```python
from build123d import *

# Parameters (mm, degrees)
SKETCH2_R               = 43.815
SKETCH2_R_2             = 40
BASE_CYLINDER_DEPTH     = 381
SKETCH3_R               = 56.35625
SKETCH3_R_2             = 40
AFT_FLANGE_DEPTH        = 9.525
SKETCH6_R               = 46.9011
SKETCH6_R_2             = 44.2849
AFT_O_RING_DEPTH        = 1.9812
SKETCH33_R              = 45.72
SKETCH33_R_2            = 43.815
CRITICALBOSS_DEPTH      = 31.75
FILLET1_R               = 2.54
BOLT_CIRCLE_D           = 4.0386
HOLE1_D                 = 2.38125
HOLE1_CBORE_D           = 4.7625
HOLE1_CBORE_DEPTH       = 4.7625
F_3_8_24_TAPPED_HOLE1_D = 8.4328
FILLET1_OF_MIRROR1_R    = 2.54


with BuildPart() as part:
    # Sketch2 → Base Cylinder (new body)
    with BuildSketch(Plane(origin=(0, 0, 0), x_dir=(1, 0, 0), z_dir=(0, 1, 0))):
        with Locations(Location((0, 0, 0), (0, 0, 270))):
            Circle(SKETCH2_R)
        with Locations(Location((0, 0, 0), (0, 0, 270))):
            Circle(SKETCH2_R_2, mode=Mode.SUBTRACT)
    extrude(amount=BASE_CYLINDER_DEPTH)

    # Sketch3 → Aft Flange (add)
    with BuildSketch(Plane.XZ):
        with Locations(Location((0, 0, 0), (0, 0, 270))):
            Circle(SKETCH3_R)
        with Locations(Location((0, 0, 0), (0, 0, 90))):
            Circle(SKETCH3_R_2, mode=Mode.SUBTRACT)
    aft_flange = extrude(amount=-AFT_FLANGE_DEPTH)

    # Sketch6 → Aft O-Ring (cut)
    with BuildSketch(Plane.XZ):
        with Locations(Location((0, 0, 0), (0, 0, 270))):
            Circle(SKETCH6_R)
        with Locations(Location((0, 0, 0), (0, 0, 270))):
            Circle(SKETCH6_R_2, mode=Mode.SUBTRACT)
    aft_o_ring = extrude(amount=-AFT_O_RING_DEPTH, mode=Mode.SUBTRACT)

    # Sketch33 → CriticalBoss (add)
    with BuildSketch(Plane(origin=(0, 9.525, 0), x_dir=(1, 0, 0), z_dir=(0, 1, 0))):
        with Locations(Location((0, 0, 0), (0, 0, 90))):
            Circle(SKETCH33_R)
        with Locations(Location((0, 0, 0), (0, 0, 270))):
            Circle(SKETCH33_R_2, mode=Mode.SUBTRACT)
    criticalboss = extrude(amount=CRITICALBOSS_DEPTH)

    # Fillet1
    # the kernel refuses this fillet: 2.54 mm, written as the material it adds along each edge
    with BuildSketch(Plane(origin=(0, 9.525, 0), x_dir=(0, 0, -1), z_dir=(1, 0, 0))) as fillet1_piece_1:
        with BuildLine():
            CenterArc((45.72 + FILLET1_R, FILLET1_R), FILLET1_R, 180, 90)
            Line((45.72, FILLET1_R), (45.72 - FILLET1_R * 0.02, FILLET1_R))
            Line((45.72 - FILLET1_R * 0.02, FILLET1_R), (45.72 - FILLET1_R * 0.02, -FILLET1_R * 0.02))
            Line((45.72 - FILLET1_R * 0.02, -FILLET1_R * 0.02), (45.72 + FILLET1_R, -FILLET1_R * 0.02))
            Line((45.72 + FILLET1_R, -FILLET1_R * 0.02), (45.72 + FILLET1_R, 0))
        make_face()
    revolve(axis=Axis((0, 9.525, 0), (0, 1, 0)))
    with BuildSketch(Plane(origin=(0, 41.275, 0), x_dir=(0, 0, 1), z_dir=(-1, 0, 0))) as fillet1_piece_2:
        with BuildLine():
            CenterArc((46.355, 2.459344425), FILLET1_R, 180, 75.522487814)
            Line((43.815, 2.459344425), (43.7642, 2.459344425))
            Line((43.7642, 2.459344425), (43.7642, 0))
            Line((43.7642, 0), (43.815, -0.0508))
            ThreePointArc((43.815, -0.0508), (44.7675, -0.0508), (45.7073, -0.049186888))
            Line((45.7073, -0.049186888), (45.72, 0))
        make_face()
    revolve(axis=Axis((0, 41.275, 0), (0, 1, 0)))

    # Bolt Circle (through all)
    with Locations(Plane(origin=(0, 0, 0), x_dir=(-1, 0, 0), z_dir=(0, -1, 0))):
        with Locations((-25.81275, -44.708994483), (-44.708994483, -25.81275), (-51.6255, 0), (-44.708994483, 25.81275), (-25.81275, 44.708994483), (0, 51.6255), (25.81275, 44.708994483), (44.708994483, 25.81275), (51.6255, 0), (44.708994483, -25.81275), (25.81275, -44.708994483), (0, -51.6255)):
            bolt_circle = Hole(BOLT_CIRCLE_D / 2)

    # Hole1 (through all)
    with Locations(Plane(origin=(0, 0, 0), x_dir=(-1, 0, 0), z_dir=(0, -1, 0))):
        with Locations((49.866403745, 13.361662613), (-49.866403745, -13.361662613)):
            hole1 = CounterBoreHole(HOLE1_D / 2, HOLE1_CBORE_D / 2, HOLE1_CBORE_DEPTH)

    # Sketch44 → 1/8 NPT Tapped ThermocoupleHole (revolve, cut)
    with BuildSketch(Plane(origin=(0, 19.05, -45.72), x_dir=(0, 1, 0), z_dir=(1, 0, 0))):
        Polygon((0, 0), (0, 14.213468714), (4.2164, 11.68), (4.2164, 6.86), (4.537404713, 6.86), (4.7428023, 0), align=None)
    revolve(axis=Axis((0, 19.05, -52.07), (0, 0, 1)), mode=Mode.SUBTRACT)

    # 3/8-24 Tapped Hole1 (through all)
    with Locations(Plane.XY.offset(45.72)):
        with Locations((0, 19.05)):
            Hole(F_3_8_24_TAPPED_HOLE1_D / 2)

    # Mirror1: Aft Flange, Aft O-Ring, CriticalBoss, Bolt Circle, Hole1 across plane
    add(aft_flange.mirror(Plane.ZX.offset(190.5)))
    add(aft_o_ring.mirror(Plane.ZX.offset(190.5)), mode=Mode.SUBTRACT)
    add(criticalboss.mirror(Plane.ZX.offset(190.5)))
    add(bolt_circle.mirror(Plane.ZX.offset(190.5)), mode=Mode.SUBTRACT)
    add(hole1.mirror(Plane.ZX.offset(190.5)), mode=Mode.SUBTRACT)

    # Fillet1 of Mirror1
    # the kernel refuses this fillet: 2.54 mm, written as the material it adds along each edge
    with BuildSketch(Plane(origin=(0, 371.475, 0), x_dir=(0, 0, -1), z_dir=(1, 0, 0))) as fillet1_of_mirror1_piece_1:
        with BuildLine():
            CenterArc((45.72 + FILLET1_OF_MIRROR1_R, -FILLET1_OF_MIRROR1_R), FILLET1_OF_MIRROR1_R, 90, 90)
            Line((45.72 + FILLET1_OF_MIRROR1_R, 0), (45.72 + FILLET1_OF_MIRROR1_R, FILLET1_OF_MIRROR1_R * 0.02))
            Line((45.72 + FILLET1_OF_MIRROR1_R, FILLET1_OF_MIRROR1_R * 0.02), (45.72 - FILLET1_OF_MIRROR1_R * 0.02, FILLET1_OF_MIRROR1_R * 0.02))
            Line((45.72 - FILLET1_OF_MIRROR1_R * 0.02, FILLET1_OF_MIRROR1_R * 0.02), (45.72 - FILLET1_OF_MIRROR1_R * 0.02, -FILLET1_OF_MIRROR1_R))
            Line((45.72 - FILLET1_OF_MIRROR1_R * 0.02, -FILLET1_OF_MIRROR1_R), (45.72, -FILLET1_OF_MIRROR1_R))
        make_face()
    revolve(axis=Axis((0, 371.475, 0), (0, 1, 0)))
    with BuildSketch(Plane(origin=(0, 339.725, 0), x_dir=(0, 0, 1), z_dir=(-1, 0, 0))) as fillet1_of_mirror1_piece_2:
        with BuildLine():
            CenterArc((46.355, -2.459344425), FILLET1_OF_MIRROR1_R, 104.477512186, 75.522487814)
            Line((45.72, 0), (45.7073, 0.049186888))
            ThreePointArc((45.7073, 0.049186888), (44.7675, 0.0508), (43.815, 0.0508))
            Line((43.815, 0.0508), (43.7642, 0))
            Line((43.7642, 0), (43.7642, -2.459344425))
            Line((43.7642, -2.459344425), (43.815, -2.459344425))
        make_face()
    revolve(axis=Axis((0, 339.725, 0), (0, 1, 0)))


solid = part.part
```
The listing builds one solid part. Answer for the finished solid, in the listing's coordinates (mm). A direction names the side the tool comes from. Coordinates: 2 decimals unless noted, no trailing zeros. Write each loop counter-clockwise with the first axis right and the second up, starting at its lowest first coordinate (ties: lowest second). Pieces come first, ordered by that corner, then holes.
Q1. The mould has two halves that part along X. Classify faces 6 (the flat face through (-23, 0, 33)), 7 (the cylindrical face through (-16.96, 380.02, -40.91)), 8 (the cylindrical face through (-21.58, 376.3, -52.06)): released by +X, released by -X, zero draft, split by the parting line, or undercut.
Returned:
face 6: zero draft
face 7: undercut
face 8: split by the parting line
Q2. Find the intervals of material crossed by line 1 along X through (y, z) = (318.5, 1); line 2 along Y through (x, z) = (-49, -17) (3 decimals); line 3 along Z through (x, y) = (-3, 326.5), in increasing order.
Returned:
line 1: x = -43.8 to -39.99, 39.99 to 43.8
line 2: y = 0 to 9.525, 371.475 to 381
line 3: z = -43.71 to -39.89, 39.89 to 43.71
Q3. Given P1, Ø2.5, axis at x = 50, z = 14, coming from the +Y side; P2, Ø8, axis at y = 291.5, z = 5, coming from the -X side; P3, Ø1.5, axis at x = 12.5, y = 241, coming from the -Z side, each flat-ended and moving along its own axis, determine where each tip first touches the part or whether it passes through.
Returned:
P1: stops at y = 376.24
P2: stops at x = -43.8
P3: stops at z = -42.21
Q4. Section B-B, the plane y = 265.5 is taken. Write down the section's boundary in (x, z) (3 decimals), then the cut area to 3 significant figures.
Returned:
outline: circle Ø87.63 at (0, 0); hole circle Ø80 at (0, 0)
area: 1,000 mm2
Q5. Which of the six approach directions +Z, -Z, +X, -X, +Y, -Y give full straight-line access (tool end or side, diameter ignored) to faces 1 (the flat face through (-35, 1.981, 28)), 2 (the flat face through (-46, 371.475, -16)), 3 (the conical face through (-1.4, 23.49, -42.77)), 4 (the flat face through (-33, 381, 34)), 5 (the cylindrical face through (-17.963, 380.023, -43.325))?
Returned:
face 1: -Y
face 2: none
face 3: -Z
face 4: +Z, -Z, +X, -X, +Y
face 5: +Y
Q6. Section A-A, the plane y = 19.05 is taken. Write down the section's boundary in (x, z).
Returned:
outline: (-4.74, -45.47) - (-4.56, -39.74) arc R40 cw to (-4.22, 39.78) - (-4.22, 45.53) arc R45.72 ccw to start; (4.22, 39.78) arc R40 cw to (4.56, -39.74) - (4.74, -45.47) arc R45.72 ccw to (4.22, 45.53) - close
